Could you check a few things on this drawing? It's one solid part, dimensions in mm from its lowest x, y, z. Give positions to 0.01 mm unless a question says otherwise; leave off trailing zeros. Order: outer loops, then holes, each group sorted by start corner. A loop starts at its lowest first (then second) coordinate and runs counter-clockwise, first axis right, second up. Notation, with made-up numbers: (71.25, 40.5) - (108.25, 40.5) arc R21 cw to (108.25, 77.5) - close; hole circle Ø8 at (-35.75, 87). An arc over 180 degrees is marked (long way). Put each result on its own line as item: value.
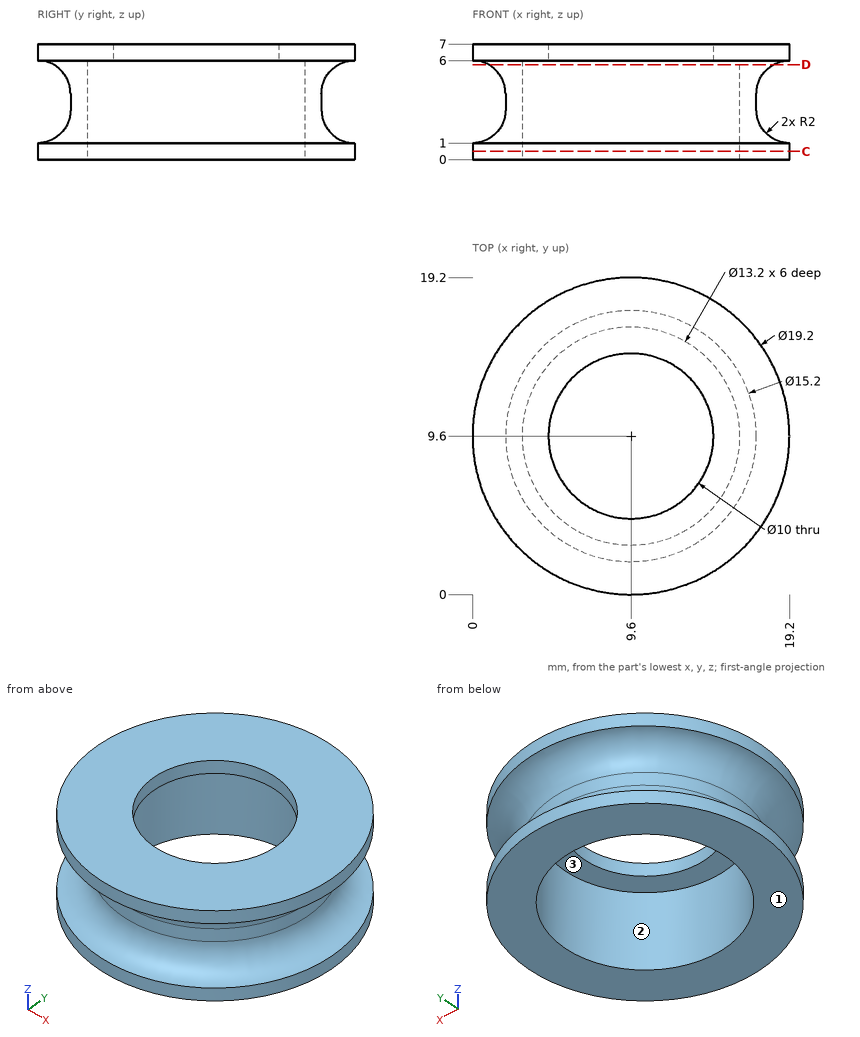
1) We'd pull the mould along Y, two halves only. Please class the marked faces 1, 2 and 3: pulls with the +Y half, pulls with the -Y half, needs draft (parallel to the pull), parting line crosses it, or undercut.
Filled in:
face 1: needs draft
face 2: undercut
face 3: undercut
2) Suppose I cut it at C-C, the plane z = 0.5. List the corners of the cut face in (x, y) for me, and give its area (3 significant figures).
Filled in:
outline: circle Ø19.2 at (9.6, 9.6); hole circle Ø13.2 at (9.6, 9.6)
area: 153 mm^2
3) I'm going to push flat-ended pins straight in: pin 1 (8 mm diameter, centred on x = 9.6, y = 9.6, fed in from -Z); pin 2 (2 mm diameter, centred on x = 5, z = 3, fed in from -Y); pin 3 (4 mm diameter, centred on y = 3, z = 5.5, fed in from -X); pin 4 (1.5 mm diameter, centred on y = 6, z = 2.5, fed in from -X). Where does each tip first touch, or does it pass through?
Filled in:
pin 1: passes through
pin 2: stops at y = 2.91
pin 3: stops at x = 1.21
pin 4: stops at x = 2.32
4) Suppose I cut it at D-D, the plane z = 5.75. List the corners of the cut face in (x, y) for me, and give its area (3 significant figures).
Filled in:
outline: circle Ø17.26 at (9.6, 9.6); hole circle Ø13.2 at (9.6, 9.6)
area: 97.2 mm^2
5) If I drill on line 1 (Y direction, x = 9.6, z = 6.5); line 2 (Z direction, x = 7.5, y = 14.75); line 3 (X direction, y = 9.5, z = 3.5), over which ranges is the centre line in solid material (lowest first)? Write a range as [from, to].
Filled in:
line 1: y = [0, 4.6], [14.6, 19.2]
line 2: z = [6, 7]
line 3: x = [2, 3], [16.2, 17.2]
